Model file for the job. Use its own axes, mm. Face numbers are marked on the shaded views. Give positions to 0.01 mm unless a question says otherwise; leave off trailing zeros. Order: outer loops, then holes, each group sorted by start corner. A loop starts at its lowest first (then second) coordinate and runs counter-clockwise, first axis right, second up. Notation, with made-up numbers: M 24,6.5 L 45,6.5 A20 cw 45,21.5 Z; hole C 87.25,12.25 d1. An arc over 180 degrees is marked long. Return JSON: item names as keys, results as strings. Group by question number.
1. Slice it at C-C on z = 8.25. List the corners of the cut face in (x, y), then the cut area to 3 significant figures.
2. Slice it at D-D on x = 25. List the corners of the cut face in (y, z), then the cut area to 3 significant figures.
3. Two-plate mould, pull along X, no slides. Class the marked faces 1, 2 and 3: released by +X, released by -X, zero draft, split by the parting line, or undercut.
4. Slice it at A-A on y = 0. List the corners of the cut face in (x, z).
5. Wall check: probe 1 along Y at (x, z) = (-23.5, 8.25); probe 2 along X at (y, z) = (24, 13.5); probe 3 along Y at (x, z) = (-25, 12). Give the ranges that are in metal, low to high. Write a range as [from, to].
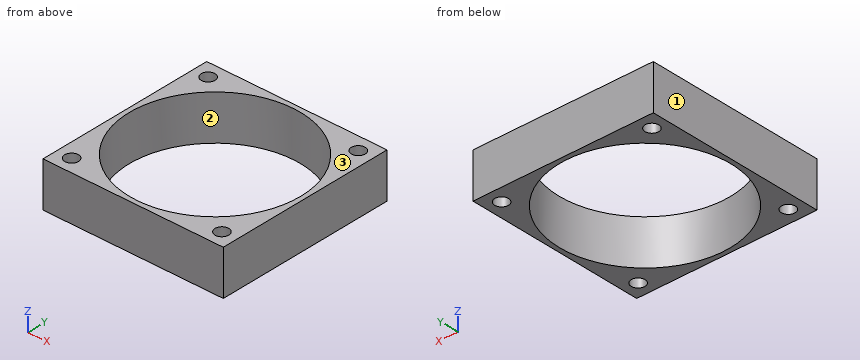
Autodesk Inventor part; units mm, degrees
ref_plane "YZ Plane" through (0, 0, 0) normal (1, 0, 0) x (0, 1, 0)
ref_plane "XZ Plane" through (0, 0, 0) normal (0, 1, 0) x (-1, 0, 0)
ref_plane "XY Plane" through (0, 0, 0) normal (0, 0, 1) x (1, 0, 0)
sketch "Sketch1" plane through (0, 0, 0) normal (0, 0, 1) x (1, 0, 0)
  line L0 (-30, -30) -> (30, -30)
  line L1 (30, -30) -> (30, 30)
  line L2 (30, 30) -> (-30, 30)
  line L3 (-30, 30) -> (-30, -30)
  line L4 (-30, -30) -> (30, 30) construction
  line L5 (30, -30) -> (-30, 30) construction
  line L6 (-25, 25) -> (25, 25) construction
  line L7 (25, 25) -> (25, -25) construction
  line L8 (25, -25) -> (-25, -25) construction
  line L9 (-25, -25) -> (-25, 25) construction
  circle A0 centre (-25, 25) radius 2.3
  circle A1 centre (25, 25) radius 2.3
  circle A2 centre (25, -25) radius 2.3
  circle A3 centre (-25, -25) radius 2.3
  circle A4 centre (0, 0) radius 28.5
  dimension "d0" = 50
  dimension "d1" = 60
  dimension "d2" = 4.6
  dimension "d3" = 57
extrude "Extrusion1" add sketch "Sketch1" along normal blind 15
properties part number "Fan" material "Silicon Nitride"
Result:
{
 "1": {"outline": "M -30,-30 L 30,-30 L 30,30 L -30,30 Z; hole C 0,0 d57; hole C -25,-25 d4.6; hole C -25,25 d4.6; hole C 25,-25 d4.6; hole C 25,25 d4.6", "area": "982 mm2"},
 "2": {"outline": "M -30,0 L -27.3,0 L -27.3,15 L -30,15 Z; M -22.7,0 L -13.68,0 L -13.68,15 L -22.7,15 Z; M 13.68,0 L 22.7,0 L 22.7,15 L 13.68,15 Z; M 27.3,0 L 30,0 L 30,15 L 27.3,15 Z", "area": "351 mm2"},
 "3": {"face 1": "released by -X", "face 2": "undercut", "face 3": "zero draft"},
 "4": {"outline": "M -30,0 L -28.5,0 L -28.5,15 L -30,15 Z; M 28.5,0 L 30,0 L 30,15 L 28.5,15 Z"},
 "5": {"probe 1": "y = [-30, -26.74], [-23.26, -16.12], [16.12, 23.26], [26.74, 30]", "probe 2": "x = [-30, -27.07], [-22.93, -15.37], [15.37, 22.93], [27.07, 30]", "probe 3": "y = [-30, -27.3], [-22.7, -13.68], [13.68, 22.7], [27.3, 30]"}
}
